```python
from build123d import *

# Parameters (mm, degrees)
SKETCH1_W           = 19.05
SKETCH1_H           = 107.95
SKETCH1_W_2         = 76.2
SKETCH1_H_2         = 19.05
BOSS_EXTRUDE1_DEPTH = 25.4


with BuildPart() as part:
    # Sketch1 → Boss-Extrude1 (new body, symmetric)
    with BuildSketch(Plane(origin=(0, 0, 0), x_dir=(1, 0, 0), z_dir=(0, 1, 0))):
        with Locations((66.675, 73.025)):
            Rectangle(SKETCH1_W, SKETCH1_H)
        with Locations((38.1, 9.525)):
            Rectangle(SKETCH1_W_2, SKETCH1_H_2)
    extrude(amount=BOSS_EXTRUDE1_DEPTH, both=True)


solid = part.part
```
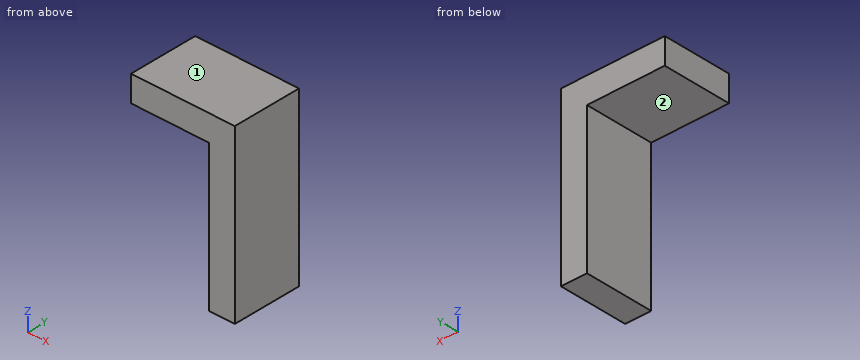
The model under review builds one solid part; all positions refer to its coordinate system, in mm. Face numbers are marked on the shaded views. A direction names the side the tool comes from. Coordinates: 2 decimals unless noted, no trailing zeros. Write each loop counter-clockwise with the first axis right and the second up, starting at its lowest first coordinate (ties: lowest second). Pieces come first, ordered by that corner, then holes.
1) To check wall thickness, follow probe 1 along X at (y, z) = (9.5, -54); probe 2 along Z at (x, y) = (31.5, -20.5). State the ranges of each line that lie inside material, in increasing order.
2) We need section C-C on x = 21. State the section outline as (y, z) points.
3) Machinability: for the marked faces 1 and 2, which of the approach directions +Z, -Z, +X, -X, +Y, -Y give a long, thin tool a straight path to every point of the face, cutting with its end or side? Answer none if there is none.
4) We need section B-B on z = -23. State the section outline as (x, y) points.
5) We need section A-A on y = 22. State the section outline as (x, z) points, then the cut area to 3 significant figures.
6) Clearance check with a flat-ended pin moving along its axis: pin 1 Ø8 at (y, z) = (-19.5, -61.5) entering from -X. State where the tip first meets the part, or that it passes through.
Answer list:
1. probe 1: x = 57.15 to 76.2
1. probe 2: z = -19.05 to 0
2. outline: (-25.4, -19.05) - (25.4, -19.05) - (25.4, 0) - (-25.4, 0) - close
3. face 1: +Z, +X, -X, +Y, -Y
3. face 2: -Z, -X, +Y, -Y
4. outline: (57.15, -25.4) - (76.2, -25.4) - (76.2, 25.4) - (57.15, 25.4) - close
5. outline: (0, -19.05) - (57.15, -19.05) - (57.15, -127) - (76.2, -127) - (76.2, 0) - (0, 0) - close
5. area: 3,510 mm2
6. pin 1: stops at x = 57.15
